Part print with two shaded views. Sizes in mm from the minimum x, y, z corner. Round coordinates to 2 decimals unless told otherwise and drop trailing zeros. Order: outer loops, then holes, each group sorted by start corner. A loop starts at its lowest first (then second) coordinate and runs counter-clockwise, first axis right, second up. Notation, with made-up numbers: (-12.5, 61) -> (11.5, 61) arc R32 cw to (11.5, 96) -> close; hole circle Ø6 at (18, 34). An arc over 180 degrees is marked (long way). Answer as a JSON object with one key per item and string values.
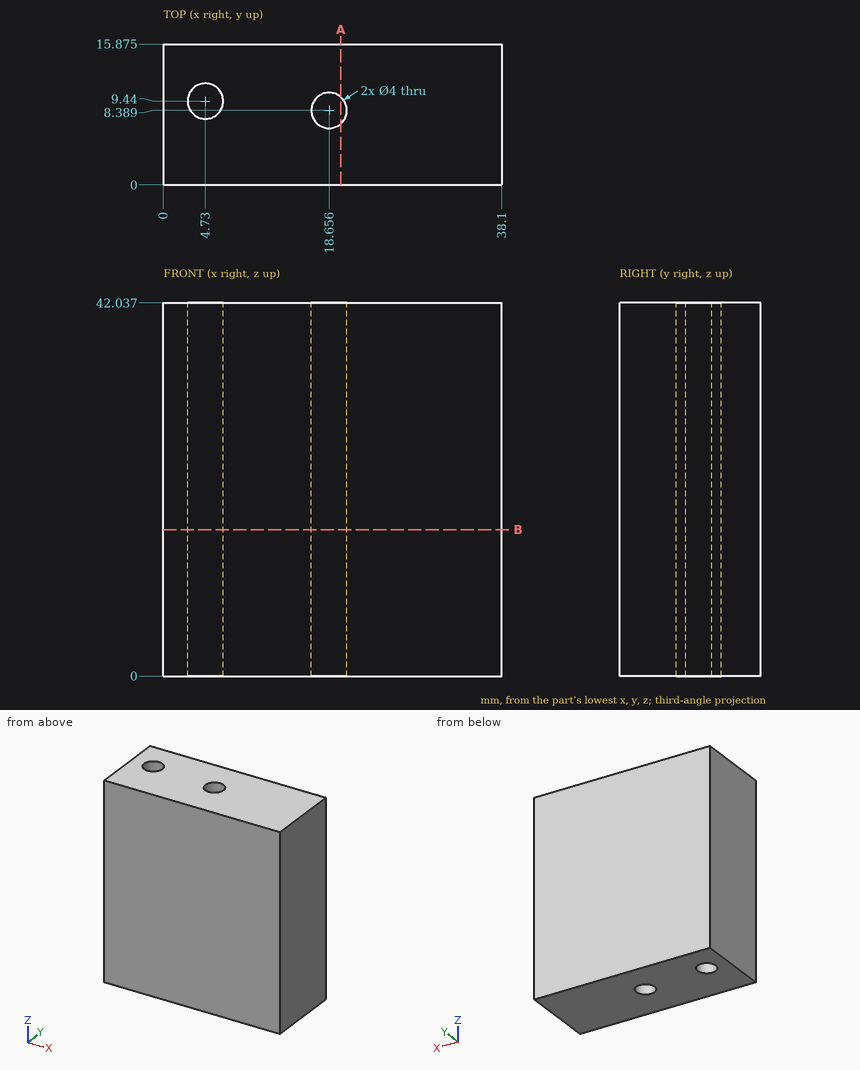
1) Probe L1, parallel to Y at x = 17, z = 33.5 (1 decimal); L2, parallel to X at y = 9.25, z = 27; L3, parallel to Y at x = 3.5, z = 6.5 (1 decimal). List the from-to ranges inside material, lowest first. Write a range as from..to.
Checked values:
{"L1": "y = 0..7.3, 9.5..15.9", "L2": "x = 0..2.74, 6.72..16.85, 20.46..38.1", "L3": "y = 0..7.9, 11..15.9"}
2) Cut at B-B, the plane z = 16.5. Give the cut face in (x, y) (1 decimal).
Checked values:
{"outline": "(0, 0) -> (38.1, 0) -> (38.1, 15.9) -> (0, 15.9) -> close; hole circle Ø4 at (4.7, 9.4); hole circle Ø4 at (18.7, 8.4)"}
3) Cut at A-A, the plane x = 20. Give the cut face in (y, z) (1 decimal), plus the area to 3 significant figures.
Checked values:
{"outline": "(0, 0) -> (6.9, 0) -> (6.9, 42) -> (0, 42) -> close; (9.9, 0) -> (15.9, 0) -> (15.9, 42) -> (9.9, 42) -> close", "area": "543 mm²"}
